Check sheet for the modelled part. Datum: model origin and axes. Units: mm. A direction names the side the tool comes from. Coordinates: 2 decimals unless noted, no trailing zeros. Loops run counter-clockwise (first coordinate to the right, second up) from the corner with the lowest first, then second, coordinate; pieces in that order, holes last. Notation, with made-up numbers: M -39.75,62.25 L -29.75,62.25 A21 cw -29.75,69.25 Z; hole C 59,8.25 d2. An arc over 180 degrees is marked long. Answer in a Markdown table with one row per item. Add a question column.
```python
from build123d import *

# Parameters (mm, degrees)
SKETCH1_W               = 166.62
SKETCH1_H               = 100.92
SKETCH1_W_2             = 79.81
SKETCH1_H_2             = 46.96
BOSS_EXTRUDE1_DEPTH     = 25
SKETCH2_W               = 166.62
SKETCH2_H               = 100.92
BOSS_EXTRUDE2_DEPTH     = 2
SKETCH3_W               = 20
SKETCH3_H               = 20
SKETCH3_W_2             = 5
SKETCH3_H_2             = 30
SKETCH3_W_3             = 25
SKETCH3_H_3             = 5
CUT_EXTRUDE1_DEPTH      = 101.557285663
SKETCH4_W               = 168.62
SKETCH4_H               = 102.92
SKETCH4_W_2             = 166.62
SKETCH4_H_2             = 100.92
BOSS_EXTRUDE3_DEPTH     = 27
FILLET1_R               = 1
SKETCH5_W               = 1
SKETCH5_H               = 5
SKETCH8_W               = 70
SKETCH8_H               = 44.022863743
CUT_EXTRUDE2_DEPTH      = 136.372458425
CUT_EXTRUDE3_DEPTH      = 2
CUT_EXTRUDE3_DEPTH_BACK = 179.061326514
SKETCH9_W               = 40
SKETCH9_H               = 21.691425142


with BuildPart() as part:
    # Sketch1 → Boss-Extrude1 (new body)
    with BuildSketch(Plane(origin=(0, 0, 0), x_dir=(1, 0, 0), z_dir=(0, 1, 0))):
        Rectangle(SKETCH1_W, SKETCH1_H)
        with Locations((41.905, 25.48)):
            Rectangle(SKETCH1_W_2, SKETCH1_H_2, mode=Mode.SUBTRACT)
        with Locations((41.905, -25.48)):
            Rectangle(SKETCH1_W_2, SKETCH1_H_2, mode=Mode.SUBTRACT)
        with Locations((-41.905, 25.48)):
            Rectangle(SKETCH1_W_2, SKETCH1_H_2, mode=Mode.SUBTRACT)
        with Locations((-41.905, -25.48)):
            Rectangle(SKETCH1_W_2, SKETCH1_H_2, mode=Mode.SUBTRACT)
    extrude(amount=BOSS_EXTRUDE1_DEPTH)

    # Sketch2 → Boss-Extrude2 (add)
    with BuildSketch(Plane.XZ):
        Rectangle(SKETCH2_W, SKETCH2_H)
    extrude(amount=BOSS_EXTRUDE2_DEPTH)

    # Sketch3 → Cut-Extrude1 (cut, through all)
    with BuildSketch(Plane(origin=(0, 0, 0), x_dir=(1, 0, 0), z_dir=(0, 1, 0))):
        Rectangle(SKETCH3_W, SKETCH3_H)
        with Locations((-79.31, 0)):
            Rectangle(SKETCH3_W_2, SKETCH3_H_2)
        with Locations((0, 46.46)):
            Rectangle(SKETCH3_W_3, SKETCH3_H_3)
        with Locations((0, -46.46)):
            Rectangle(SKETCH3_W_3, SKETCH3_H_3)
        with Locations((79.31, 0)):
            Rectangle(SKETCH3_W_2, SKETCH3_H_2)
    extrude(amount=CUT_EXTRUDE1_DEPTH, mode=Mode.SUBTRACT)

    # Sketch4 → Boss-Extrude3 (add)
    with BuildSketch(Plane.XZ.offset(2)):
        Rectangle(SKETCH4_W, SKETCH4_H)
        Rectangle(SKETCH4_W_2, SKETCH4_H_2, mode=Mode.SUBTRACT)
    extrude(amount=-BOSS_EXTRUDE3_DEPTH)

    # Fillet1
    fillet1_edges = [part.edges().sort_by_distance(p)[0] for p in [
        (-43.405, 0, 2),
        (43.405, 0, -2),
        (43.405, 25, -2),
        (-43.405, 25, 2),
        (2, 25, 26.98),
        (-2, 25, -26.98),
        (-10, 12.5, -2),
        (-10, 0, 0),
        (-10, 12.5, 2),
        (0, 0, 10),
        (2, 12.5, 10),
        (-2, 12.5, 10),
        (10, 12.5, 2),
        (10, 0, 0),
        (10, 12.5, -2),
        (0, 0, -10),
        (-2, 12.5, -10),
        (2, 12.5, -10),
        (-43.405, 0, -2),
        (-43.405, 25, -2),
        (-76.81, 0, 0),
        (-76.81, 12.5, -2),
        (-76.81, 12.5, 2),
        (2, 0, -26.98),
        (2, 25, -26.98),
        (-2, 12.5, -43.96),
        (0, 0, -43.96),
        (2, 12.5, -43.96),
        (-2, 0, 26.98),
        (-2, 25, 26.98),
        (2, 12.5, 43.96),
        (0, 0, 43.96),
        (-2, 12.5, 43.96),
        (43.405, 0, 2),
        (43.405, 25, 2),
        (76.81, 0, 0),
        (76.81, 12.5, 2),
        (76.81, 12.5, -2),
        (-2, 0, -26.98),
        (2, 0, 26.98),
    ]]
    fillet(fillet1_edges, radius=FILLET1_R)

    # Cut-Sweep1: sweep along a path in Sketch7
    with BuildLine(Plane(origin=(0, 25, 0), x_dir=(1, 0, 0), z_dir=(0, 1, 0))) as cut_sweep1_path:
        Line((-84.31, -51.46), (84.31, -51.46))
        Line((84.31, -51.46), (84.31, 51.46))
        Line((84.31, 51.46), (-84.31, 51.46))
        Line((-84.31, 51.46), (-84.31, -51.46))
    # Sketch5 → Cut-Sweep1 (sweep, cut)
    with BuildSketch(Plane(origin=(84.31, 0, 0), x_dir=(0, 0, -1), z_dir=(1, 0, 0))):
        with Locations((-50.96, 22.5)):
            Rectangle(SKETCH5_W, SKETCH5_H)
    sweep(path=cut_sweep1_path.line, transition=Transition.RIGHT, mode=Mode.SUBTRACT)

    # Sketch8 → Cut-Extrude2 (cut, through all)
    with BuildSketch(Plane.XY.offset(51.46)):
        with Locations((-42.31, 30.011431872)):
            Rectangle(SKETCH8_W, SKETCH8_H)
        with Locations((42.31, 30.011431872)):
            Rectangle(SKETCH8_W, SKETCH8_H)
    extrude(amount=-CUT_EXTRUDE2_DEPTH, mode=Mode.SUBTRACT)

    # Sketch9 → Cut-Extrude3 (cut, two sides: drawn at the far end of the back side and taken through both)
    with BuildSketch(Plane(origin=(84.31, 0, 0), x_dir=(0, 0, -1), z_dir=(1, 0, 0)).offset(-CUT_EXTRUDE3_DEPTH_BACK)):
        with Locations((-24.46, 18.845712571)):
            Rectangle(SKETCH9_W, SKETCH9_H)
        with Locations((24.46, 18.845712571)):
            Rectangle(SKETCH9_W, SKETCH9_H)
    extrude(amount=CUT_EXTRUDE3_DEPTH + CUT_EXTRUDE3_DEPTH_BACK, mode=Mode.SUBTRACT)


solid = part.part
```
Q1. Cross-section at C-C (x = -63). Record the cut outline in (y, z), plus the area to 3 significant figures.
Q2. Go/stop test with flat-tipped pins: pin 1 (8 mm diameter, centred on x = -36.5, z = -6.5, fed in from +Y); pin 2 (3 mm diameter, centred on x = 28, z = 0.5, fed in from +Y); pin 3 (1.5 mm diameter, centred on x = -21, z = 9.5, fed in from +Y). Record where each tip stops, or that it passes through.
Q3. Thickness scan on L1, parallel to Z at x = 66.5, y = 2; L2, parallel to X at y = 1, z = 23; L3, parallel to X at y = 9.25, z = -3.5. Record the ranges inside material, lowest first.
Q4. Cross-section at A-A (y = 23.25). Count the separate pieces of the cut face and the enclosed holes in it, plus the area to 3 significant figures.
Q5. Mould release check, pull along X, two halves, no side actions. Record for faces 6 (the face through (43, 4, -2)), 7 (the face through (0, 8, 27)), 8 (the face through (84.31, 6, -1)): released by +X, released by -X, zero draft, split by the parting line, or undercut.
Q6. Cross-section at B-B (z = -21.5). Record the cut outline in (x, y), plus the area to 3 significant figures.
Q7. Access from +Z, -Z, +X, -X, +Y, -Y to the whole of each face (thin tool, end or side, straight path). Record for faces 1 (the face through (-83.31, 22, 48)), 2 (the face through (0, 22, -50.46)), 3 (the face through (83.31, 22, 47)), 4 (the face through (-1, 0, 1)), 5 (the face through (0, 22, 50.46)).
Answer key:
| question | item | result |
|---|---|---|
| 1 | outline | M -2,-51.46 L 8,-51.46 L 8,-48.96 L 0,-48.96 L 0,-3 A1 cw 1,-2 L 8,-2 L 8,2 L 1,2 A1 cw 0,3 L 0,48.96 L 8,48.96 L 8,51.46 L -2,51.46 Z |
| 1 | area | 278 mm^2 |
| 2 | pin 1 | y = 0.13 |
| 2 | pin 2 | y = 8 |
| 2 | pin 3 | y = 0 |
| 3 | L1 | -51.46 to -48.96, -2 to 2, 48.96 to 51.46 |
| 3 | L2 | -84.31 to -81.81, -2 to 2, 81.81 to 84.31 |
| 3 | L3 | -84.31 to -81.81, 81.81 to 84.31 |
| 4 | separate pieces | 8 |
| 4 | enclosed holes | 0 |
| 4 | area | 134 mm^2 |
| 5 | face 6 | undercut |
| 5 | face 7 | zero draft |
| 5 | face 8 | released by +X |
| 6 | outline | M -84.31,-2 L 84.31,-2 L 84.31,8 L 81.81,8 L 81.81,0 L 3,0 A1 cw 2,1 L 2,8 L -2,8 L -2,1 A1 cw -3,0 L -81.81,0 L -81.81,8 L -84.31,8 Z |
| 6 | area | 410 mm^2 |
| 7 | face 1 | +Z, -Z, -X, +Y |
| 7 | face 2 | -Z, +X, -X, +Y |
| 7 | face 3 | +Z, -Z, +X, +Y |
| 7 | face 4 | +Y |
| 7 | face 5 | +Z, +X, -X, +Y |
